For this review, take the finished solid that the model builds, in its own axes (mm). A direction names the side the tool comes from. Coordinates: 2 decimals unless noted, no trailing zeros. Write each loop counter-clockwise with the first axis right and the second up, starting at its lowest first coordinate (ties: lowest second). Pieces come first, ordered by that corner, then holes.
```python
from build123d import *

# Parameters (mm, degrees)
F0_R           = 4.55
F1_DEPTH       = 7
F3_D           = 2.5
F3_CBORE_D     = 5
F3_CBORE_DEPTH = 5
F4_D           = 2.7
F4_CBORE_D     = 6
F4_CBORE_DEPTH = 2
F5_R           = 25


with BuildPart() as f1:
    # F0 (on Front) → F1 (new body)
    with BuildSketch(Plane.XZ):
        with BuildLine():
            ThreePointArc((4.3861063064, -13.0844209451), (11.2019700729, -8.0595202392), (13.8, 0))
            ThreePointArc((13.8, 0), (11.2019700729, 8.0595202392), (4.3861063064, 13.0844209451))
            ThreePointArc((4.3861063064, 13.0844209451), (-13.8, 0), (4.3861063064, -13.0844209451))
        make_face()
        Circle(F0_R, mode=Mode.SUBTRACT)
        with BuildLine():
            ThreePointArc((4.3861063064, 13.0844209451), (11.2019700729, 8.0595202392), (13.8, 0))
            ThreePointArc((13.8, 0), (11.2019700729, -8.0595202392), (4.3861063064, -13.0844209451))
            ThreePointArc((4.3861063064, -13.0844209451), (25.3974589974, -9.5066550069), (46.5, -12.5))
            Line((46.5, -12.5), (51.5, -12.5))
            Line((51.5, -12.5), (51.5, 12.5))
            Line((51.5, 12.5), (46.5, 12.5))
            ThreePointArc((46.5, 12.5), (25.3974589974, 9.5066550069), (4.3861063064, 13.0844209451))
        make_face()
    extrude(amount=F1_DEPTH)

    # F3 (through all)
    with Locations(Plane(origin=(0, 0, 0), x_dir=(1, 0, 0), z_dir=(0, 1, 0))):
        with Locations((-2.95, -5.1095498823), (-2.95, 5.1095498823), (5.9, 0)):
            CounterBoreHole(F3_D / 2, F3_CBORE_D / 2, F3_CBORE_DEPTH)

    # F4 (through all)
    with Locations(Plane.XZ.offset(7)):
        with Locations((49, 7.5), (49, -7.5)):
            CounterBoreHole(F4_D / 2, F4_CBORE_D / 2, F4_CBORE_DEPTH)

    # F5
    f5_edges = [f1.edges().sort_by_distance(p)[0] for p in [
        (46.5, -3.5, 12.5),
        (46.5, -3.5, -12.5),
    ]]
    fillet(f5_edges, radius=F5_R)


solid = f1.part
```
Q1. Add section A-A (z = 0). State the section outline as (x, y) points.
Ans:
outline: (-13.8, -7) - (-4.55, -7) - (-4.55, 0) - (-13.8, 0) - close; (4.55, -7) - (4.65, -7) - (4.65, -5) - (4.55, -5) - close; (7.15, -7) - (51.5, -7) - (51.5, 0) - (8.4, 0) - (8.4, -5) - (7.15, -5) - close
Q2. Draft analysis for pull direction Z (two halves, no side actions). For faces 5 (the flat face through (18, 0, 0)), 6 (the flat face through (51, -3, -12.5)), 7 (the flat face through (7, -5, -1)), state which applies: +Z half, -Z half, draft (parallel to the pull), parting line (faces both ways), or undercut.
Ans:
face 5: draft
face 6: -Z half
face 7: undercut
Q3. Add section B-B (x = -2.95). State the section outline as (y, z) points.
Ans:
outline: (-7, -13.48) - (0, -13.48) - (0, -7.61) - (-5, -7.61) - (-5, -6.36) - (-7, -6.36) - close; (-7, -3.86) - (-5, -3.86) - (-5, -3.46) - (-7, -3.46) - close; (-7, 3.46) - (-5, 3.46) - (-5, 3.86) - (-7, 3.86) - close; (-7, 6.36) - (-5, 6.36) - (-5, 7.61) - (0, 7.61) - (0, 13.48) - (-7, 13.48) - close
Q4. Clearance check with flat-ended pins moving along their axes: pin 1 Ø4 at (x, z) = (5.9, 0) entering from +Y; pin 2 Ø3 at (x, z) = (48.5, -8) entering from -Y; pin 3 Ø2 at (x, y) = (26, -2.5) entering from -Z. State where each tip first meets the part, or that it passes through.
Ans:
pin 1: stops at y = -5
pin 2: stops at y = -5
pin 3: stops at z = -9.51
Q5. Add section D-D (y = -1.5). State the section outline as (x, z) points.
Ans:
outline: (4.39, -13.08) arc R69.13 cw to (43.67, -11.7) arc R25 ccw to (49.93, -12.5) - (51.5, -12.5) - (51.5, 12.5) - (49.93, 12.5) arc R25 ccw to (43.67, 11.7) arc R69.13 cw to (4.39, 13.08) arc R13.8 ccw (long way) to start; hole (-3.65, -2.71) arc R2.5 ccw (long way) to (-0.52, -4.52) arc R4.55 ccw to (4.17, -1.81) arc R2.5 ccw (long way) to (4.17, 1.81) arc R4.55 ccw to (-0.52, 4.52) arc R2.5 ccw (long way) to (-3.65, 2.71) arc R4.55 ccw to start; hole circle Ø2.7 at (49, -7.5); hole circle Ø2.7 at (49, 7.5)
Q6. For probe 1 along Z at (x, y) = (49, -5.85); probe 2 along X at (y, z) = (-6.5, 5.5); probe 3 along Z at (x, y) = (9, -2), list the stretches that pass through material, from the lowest coordinate up.
Ans:
probe 1: z = -12.48 to -10.5, -4.5 to 4.5, 10.5 to 12.48
probe 2: x = -12.66 to -4.14, -1.76 to 46.76, 51.24 to 51.5
probe 3: z = -11.71 to 11.71
Q7. Tool access review of faces 1 (the flat face through (49, -5, 9)), 2 (the cylindrical face through (46.731, -3.549, 12.294)), 3 (the cylindrical face through (46.731, -3.549, -12.294)), 4 (the cylindrical face through (8.4, -2.5, 0.1)): name each direction out of +Z, -Z, +X, -X, +Y, -Y from which nothing blocks a thin tool from reaching the whole face with its end or side.
Ans:
face 1: -Y
face 2: +Z, +Y, -Y
face 3: -Z, +Y, -Y
face 4: +Y
Q8. Add section C-C (x = 49). State the section outline as (y, z) points, then the cut area to 3 significant figures.
Ans:
outline: (-7, -12.48) - (0, -12.48) - (0, -8.85) - (-5, -8.85) - (-5, -10.5) - (-7, -10.5) - close; (-7, -4.5) - (-5, -4.5) - (-5, -6.15) - (0, -6.15) - (0, 6.15) - (-5, 6.15) - (-5, 4.5) - (-7, 4.5) - close; (-7, 10.5) - (-5, 10.5) - (-5, 8.85) - (0, 8.85) - (0, 12.48) - (-7, 12.48) - close
area: 124 mm2
